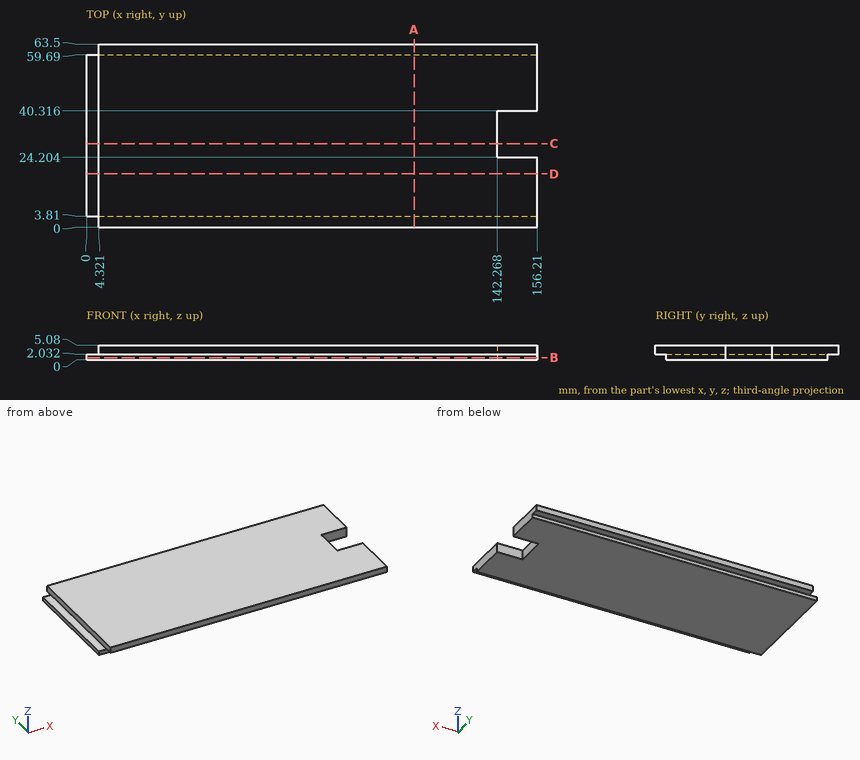
The drawing under review shows one solid part. Ordinate dimensions are in mm from its lowest x, y, z. Coordinates: 2 decimals unless noted, no trailing zeros. Write each loop counter-clockwise with the first axis right and the second up, starting at its lowest first coordinate (ties: lowest second). Pieces come first, ordered by that corner, then holes.
1) Add section A-A (x = 113.5). Write out the cut boundary in (y, z).
2) Add section C-C (y = 29). Write out the cut boundary in (x, z).
3) Insertion check: pin 1 (5 mm diameter, centred on x = 1.5, y = 36.5, fed in from +Z); pin 2 (2 mm diameter, centred on x = 99.5, z = 0.5, fed in from +Y); pin 3 (1.9 mm diameter, centred on x = 99.5, y = 61.5, fed in from -Z). Each pin has a flat end and moves straight along its axis. Give the tip position at first contact, or say it passes through.
4) Add section D-D (y = 18.5). Write out the cut boundary in (x, z).
5) Add section B-B (z = 0.8). Write out the cut boundary in (x, y) (1 decimal), plus the area to 3 significant figures.
6) To check wall thickness, follow L1, parallel to Y at x = 149.5, z = 1 (1 decimal); L2, parallel to X at y = 57, z = 4.3; L3, parallel to X at y = 25.5, z = 1.9. State the ranges of each line that lie inside material, in increasing order.
Check result:
1. outline: (0, 2.03) - (3.81, 2.03) - (3.81, 0) - (59.69, 0) - (59.69, 2.03) - (63.5, 2.03) - (63.5, 5.08) - (0, 5.08) - close
2. outline: (0, 0) - (142.27, 0) - (142.27, 5.08) - (4.32, 5.08) - (4.32, 2.03) - (0, 2.03) - close
3. pin 1: stops at z = 2.03
3. pin 2: stops at y = 59.69
3. pin 3: stops at z = 2.03
4. outline: (0, 0) - (156.21, 0) - (156.21, 5.08) - (4.32, 5.08) - (4.32, 2.03) - (0, 2.03) - close
5. outline: (0, 3.8) - (156.2, 3.8) - (156.2, 24.2) - (142.3, 24.2) - (142.3, 40.3) - (156.2, 40.3) - (156.2, 59.7) - (0, 59.7) - close
5. area: 8,500 mm2
6. L1: y = 3.8 to 24.2, 40.3 to 59.7
6. L2: x = 4.32 to 156.21
6. L3: x = 0 to 142.27
